For this review, take the finished solid that the model builds, in its own axes (mm). Face numbers are marked on the shaded views. A direction names the side the tool comes from. Give positions to 0.01 mm unless a question says otherwise; leave off trailing zeros. Loops run counter-clockwise (first coordinate to the right, second up) from the corner with the lowest first, then second, coordinate; pieces in that order, holes last.
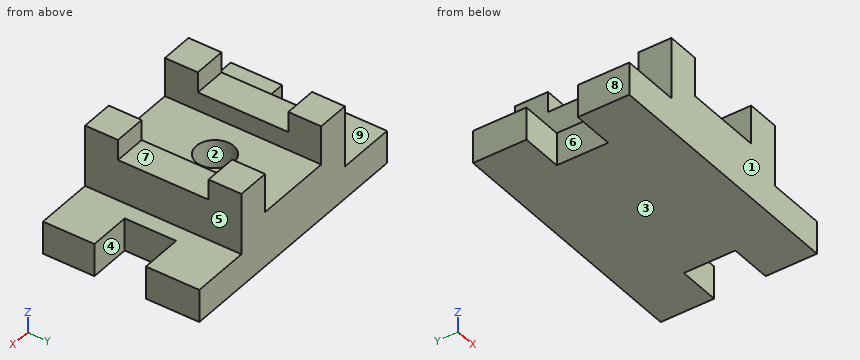
```python
from build123d import *

# Parameters (mm, degrees)
F0_W      = 129.032
F0_H      = 77.216
F1_DEPTH  = 46.736
F2_W      = 28.956
F2_H      = 77.216
F3_DEPTH  = 30.48
F4_DEPTH  = 30.48
F5_W      = 38.608
F5_H      = 77.216
F6_DEPTH  = 19.304
F7_W      = 16.256
F7_H      = 44.704
F8_DEPTH  = 10.16
F9_W      = 16.256
F9_H      = 44.704
F10_DEPTH = 10.16
F11_W     = 20.828
F11_H     = 25.4
F12_DEPTH = 16.256
F13_W     = 20.828
F13_H     = 25.4
F14_DEPTH = 16.256
F15_R     = 9.294424
F16_DEPTH = 16.256


with BuildPart() as f1:
    # F0 (on Top) → F1 (new body)
    with BuildSketch(Plane.XY):
        with Locations((1.073599, 0.463698)):
            Rectangle(F0_W, F0_H)
    extrude(amount=F1_DEPTH)

    # F2 (on face) → F3 (cut)
    with BuildSketch(Plane.XY.offset(46.736)):
        with Locations((-48.964401, 0.463698)):
            Rectangle(F2_W, F2_H)
    extrude(amount=-F3_DEPTH, mode=Mode.SUBTRACT)

    # F2 (on face) → F4 (cut)
    with BuildSketch(Plane.XY.offset(46.736)):
        with Locations((51.111599, 0.463698)):
            Rectangle(F2_W, F2_H)
    extrude(amount=-F4_DEPTH, mode=Mode.SUBTRACT)

    # F5 (on face) → F6 (cut)
    with BuildSketch(Plane.XY.offset(46.736)):
        with Locations((1.073599, 0.463698)):
            Rectangle(F5_W, F5_H)
    extrude(amount=-F6_DEPTH, mode=Mode.SUBTRACT)

    # F7 (on face) → F8 (cut)
    with BuildSketch(Plane.XY.offset(46.736)):
        with Locations((-26.358401, 0.463698)):
            Rectangle(F7_W, F7_H)
    extrude(amount=-F8_DEPTH, mode=Mode.SUBTRACT)

    # F9 (on face) → F10 (cut)
    with BuildSketch(Plane.XY.offset(46.736)):
        with Locations((28.505599, 0.463698)):
            Rectangle(F9_W, F9_H)
    extrude(amount=-F10_DEPTH, mode=Mode.SUBTRACT)

    # F11 (on face) → F12 (cut)
    with BuildSketch(Plane.XY.offset(16.256)):
        with Locations((55.175599, -0.044302)):
            Rectangle(F11_W, F11_H)
    extrude(amount=-F12_DEPTH, mode=Mode.SUBTRACT)

    # F13 (on face) → F14 (cut)
    with BuildSketch(Plane.XY.offset(16.256)):
        with Locations((-53.028401, -0.044302)):
            Rectangle(F13_W, F13_H)
    extrude(amount=-F14_DEPTH, mode=Mode.SUBTRACT)

    # F15 (on face) → F16 (cut)
    with BuildSketch(Plane.XY.offset(27.432)):
        with Locations((1.073599, 0.463698)):
            Circle(F15_R)
    extrude(amount=-F16_DEPTH, mode=Mode.SUBTRACT)


solid = f1.part
```
Item 1: Clearance check with flat-ended pins moving along their axes: pin 1 Ø5 at (x, y) = (-28, -7.5) entering from +Z; pin 2 Ø15 at (x, y) = (1.07, 0.46) entering from +Z; pin 3 Ø8.5 at (x, y) = (46, -10.5) entering from +Z. State where each tip first meets the part, or that it passes through.
Answer:
pin 1: stops at z = 36.58
pin 2: stops at z = 11.18
pin 3: stops at z = 16.26
Item 2: Take a section at C-C on y = 15. Give the boundary of the cut face in (x, z), and give its area (3 significant figures).
Answer:
outline: (-63.44, 0) - (65.59, 0) - (65.59, 16.26) - (36.63, 16.26) - (36.63, 36.58) - (20.38, 36.58) - (20.38, 27.43) - (-18.23, 27.43) - (-18.23, 36.58) - (-34.49, 36.58) - (-34.49, 16.26) - (-63.44, 16.26) - close
area: 3,190 mm2
Item 3: Take a section at A-A on z = 43. Give the boundary of the cut face in (x, y), and give its area (3 significant figures).
Answer:
outline: (-34.49, -38.14) - (-18.23, -38.14) - (-18.23, -21.89) - (-34.49, -21.89) - close; (-34.49, 22.82) - (-18.23, 22.82) - (-18.23, 39.07) - (-34.49, 39.07) - close; (20.38, -38.14) - (36.63, -38.14) - (36.63, -21.89) - (20.38, -21.89) - close; (20.38, 22.82) - (36.63, 22.82) - (36.63, 39.07) - (20.38, 39.07) - close
area: 1,060 mm2
Item 4: Tool access review of the marked faces 5, 6, 7, 8 and 9: name each direction out of +Z, -Z, +X, -X, +Y, -Y from which nothing blocks a thin tool from reaching the whole face with its end or side.
Answer:
face 5: +Z, +X, +Y, -Y
face 6: +Z, -Z, -X
face 7: +Z, +X, -X
face 8: +Z, -Z, -X, +Y, -Y
face 9: +Z, -X, +Y, -Y
Item 5: The part is to be moulded in two halves that separate along Y. For the marked faces 1, 2, 3 and 4, say which applies: released by +Y, released by -Y, zero draft, split by the parting line, or undercut.
Answer:
face 1: released by -Y
face 2: undercut
face 3: zero draft
face 4: undercut
Item 6: Take a section at D-D on z = 30.5. Give the boundary of the cut face in (x, y).
Answer:
outline: (-34.49, -38.14) - (-18.23, -38.14) - (-18.23, 39.07) - (-34.49, 39.07) - close; (20.38, -38.14) - (36.63, -38.14) - (36.63, 39.07) - (20.38, 39.07) - close
Item 7: For L1, parallel to X at y = 25, z = 36.5; L2, parallel to Y at x = 50, z = 4; L3, parallel to Z at x = -42.5, y = 27.5, list the stretches that pass through material, from the lowest coordinate up.
Answer:
L1: x = -34.49 to -18.23, 20.38 to 36.63
L2: y = -38.14 to -12.74, 12.66 to 39.07
L3: z = 0 to 16.26
Item 8: Take a section at B-B on x = 48.5. Give the boundary of the cut face in (y, z), and give its area (3 significant figures).
Answer:
outline: (-38.14, 0) - (-12.74, 0) - (-12.74, 16.26) - (-38.14, 16.26) - close; (12.66, 0) - (39.07, 0) - (39.07, 16.26) - (12.66, 16.26) - close
area: 842 mm2
